```python
from build123d import *

# Parameters (mm, degrees)
SKETCH_1_R      = 65
EXTRUDE_1_DEPTH = 3
SKETCH_2_W      = 70
SKETCH_2_H      = 70
EXTRUDE_2_DEPTH = 120
SHELL_2_T       = -7


with BuildPart() as part:
    # 草图1 → 凸台-拉伸1 (new body)
    with BuildSketch(Plane(origin=(0, 0, 0), x_dir=(1, 0, 0), z_dir=(0, 1, 0))):
        with Locations(Location((0, 0, 0), (0, 0, 270))):
            Circle(SKETCH_1_R)
    extrude(amount=EXTRUDE_1_DEPTH)

    # 草图2 → 凸台-拉伸2 (add)
    with BuildSketch(Plane(origin=(0, 3, 0), x_dir=(1, 0, 0), z_dir=(0, 1, 0))):
        Rectangle(SKETCH_2_W, SKETCH_2_H)
    extrude(amount=EXTRUDE_2_DEPTH)

    # 抽壳2
    shell_2_openings = [part.faces().sort_by_distance(p)[0] for p in [
        (0, 123, 0),
    ]]
    offset(amount=SHELL_2_T, openings=shell_2_openings, kind=Kind.INTERSECTION)


solid = part.part
```
The listing builds one solid part. Answer for the finished solid, in the listing's coordinates (mm). A direction names the side the tool comes from. Coordinates: 2 decimals unless noted, no trailing zeros. Order: outer loops, then holes, each group sorted by start corner. A loop starts at its lowest first (then second) coordinate and runs counter-clockwise, first axis right, second up. Notation, with made-up numbers: M -33,63.5 L -27,63.5 A33 ccw -27,99.5 Z; hole C -15.75,-37 d10. An arc over 180 degrees is marked long. Answer as a JSON object with one key per item and string values. Group by question number.
1. Determine the mould class of faces 1 (the flat face through (1, 3, 42)), 2 (the flat face through (-28, 64, 0)), 3 (the cylindrical face through (19.52, 1.48, 62)), 4 (the flat face through (35, 62, 0)) for opening direction X: released by +X, released by -X, zero draft, split by the parting line, or undercut.
2. Flat-ended cylindrical pins translate along their axes: P1, Ø5, axis at x = 20.5, y = 89, coming from the +Z side; P2, Ø1.5, axis at x = 36.5, z = 26, coming from the +Y side; P3, Ø5, axis at y = 107, z = 24.5, coming from the +X side. Find the tip coordinate at first contact, or state that the pin passes through.
3. Straight lines are drawn through the part: line 1 (Z direction, x = 23, y = 107); line 2 (X direction, y = 106, z = -31). For each, find the intervals that lie inside material, in ascending order.
4. Section D-D on z = -52.5 is taken. Write down the section's boundary in (x, y).
5. Section C-C on x = -6.5 is taken. Write down the section's boundary in (y, z), then the cut area to 3 significant figures.
6. A tool of negligible diameter and unlimited length cuts with its end or side. For faces 5 (the flat face through (0, 62, -35)), 6 (the flat face through (-35, 62, 0)), 7 (the flat face through (0, 62, 35)), 8 (the flat face through (1, 0, -1)), 9 (the flat face through (28, 64, 0)), from which of +Z, -Z, +X, -X, +Y, -Y can it reach the whole face along a straight path? Write none if from no direction.
7. Section B-B on y = 111 is taken. Write down the section's boundary in (x, z).
8. Section A-A on z = 0 is taken. Write down the section's boundary in (x, y), then the cut area to 3 significant figures.
Values follow:
{
 "1": {"face 1": "zero draft", "face 2": "undercut", "face 3": "split by the parting line", "face 4": "released by +X"},
 "2": {"P1": "z = 35", "P2": "y = 3", "P3": "x = 35"},
 "3": {"line 1": "-35 to -28, 28 to 35", "line 2": "-35 to 35"},
 "4": {"outline": "M -38.32,0 L 38.32,0 L 38.32,3 L -38.32,3 Z"},
 "5": {"outline": "M 0,-64.67 L 3,-64.67 L 3,-35 L 123,-35 L 123,-28 L 7,-28 L 7,28 L 123,28 L 123,35 L 3,35 L 3,64.67 L 0,64.67 Z", "area": "2,290 mm2"},
 "6": {"face 5": "-Z, +X, -X, +Y", "face 6": "+Z, -Z, -X, +Y", "face 7": "+Z, +X, -X, +Y", "face 8": "+Z, -Z, +X, -X, -Y", "face 9": "+Y"},
 "7": {"outline": "M -35,-35 L 35,-35 L 35,35 L -35,35 Z; hole M -28,-28 L 28,-28 L 28,28 L -28,28 Z"},
 "8": {"outline": "M -65,0 L 65,0 L 65,3 L 35,3 L 35,123 L 28,123 L 28,7 L -28,7 L -28,123 L -35,123 L -35,3 L -65,3 Z", "area": "2,290 mm2"}
}
